The listing builds one solid part. Answer for the finished solid, in the listing's coordinates (mm). Face numbers are marked on the shaded views. A direction names the side the tool comes from. Coordinates: 2 decimals unless noted, no trailing zeros. Loops run counter-clockwise (first coordinate to the right, second up) from the corner with the lowest first, then second, coordinate; pieces in that order, holes last. Notation, with made-up numbers: (-17.75, -4.75) - (32.25, -4.75) arc R9 cw to (32.25, 8.25) - close; hole circle Ø4 at (6.5, 50.25). An arc over 180 degrees is marked (long way). Return JSON: item names as keys, results as strings. Group by question number.
1. Section C-C (y = -2.5) is taken. Write down the section's boundary in (x, z), and give its area (3 significant figures).
2. The mould has two halves that part along Z. Classify the marked faces 1, 2 and 3: pulls with the +Z half, pulls with the -Z half, needs draft (parallel to the pull), parting line crosses it, or undercut.
3. Section A-A (y = -27) is taken. Write down the section's boundary in (x, z), and give its area (3 significant figures).
4. Section D-D (y = 5.5) is taken. Write down the section's boundary in (x, z), and give its area (3 significant figures).
5. Find the intervals of material crossed by line 1 along Z through (x, y) = (0, -26.25); line 2 along X through (y, z) = (-17, 0); line 3 along Y through (x, z) = (0, -0.5), in increasing order.
6. Each of these flat-tipped pins is pushed along its axis until it touches: P1, Ø6, axis at x = 4.5, z = 7, coming from the +Y side; P2, Ø4, axis at x = -6.5, z = 8, coming from the +Y side; P3, Ø2, axis at x = -6.5, z = -5, coming from the +Y side. Where does it stop, or does it pass through?
7. Section B-B (x = 0) is taken. Write down the section's boundary in (y, z).
8. Which of the six approach directions +Z, -Z, +X, -X, +Y, -Y give full straight-line access (tool end or side, diameter ignored) to the marked faces 4, 5 and 6?
```python
from build123d import *

# Parameters (mm, degrees)
CROQUIS1_R              = 6.5
SALIENTE_EXTRUIR1_DEPTH = 12.5
CROQUIS3_W              = 19
CROQUIS3_H              = 25
CROQUIS3_R              = 6.5
SALIENTE_EXTRUIR2_DEPTH = 25
CROQUIS8_W              = 2
CROQUIS8_H              = 5


with BuildPart() as part:
    # Croquis1 → Saliente-Extruir1 (new body, symmetric)
    with BuildSketch(Plane.XY):
        with BuildLine():
            Line((-9.5, -10), (9.5, -10))
            Line((9.5, -10), (9.5, 0))
            ThreePointArc((9.5, 0), (0, 9.5), (-9.5, 0))
            Line((-9.5, 0), (-9.5, -10))
        make_face()
        Circle(CROQUIS1_R, mode=Mode.SUBTRACT)
    extrude(amount=SALIENTE_EXTRUIR1_DEPTH, both=True)

    # Croquis3 → Saliente-Extruir2 (add)
    with BuildSketch(Plane(origin=(0, -10, 0), x_dir=(-1, 0, 0), z_dir=(0, -1, 0))):
        Rectangle(CROQUIS3_W, CROQUIS3_H)
        Circle(CROQUIS3_R, mode=Mode.SUBTRACT)
    extrude(amount=SALIENTE_EXTRUIR2_DEPTH)

    # Croquis8 → Cortar-Revolución1 (revolve, cut)
    with BuildSketch(Plane.XY):
        Polygon((-11.434596491, -17.257283371), (-11.434596491, -12.257283371), (-9.5, -11.75), (-9.5, -16.75), align=None)
        with Locations((-10.5, -27.25)):
            Rectangle(CROQUIS8_W, CROQUIS8_H)
    revolve(axis=Axis((0, -6.5, 0), (0, -1, 0)), mode=Mode.SUBTRACT)


solid = part.part
```
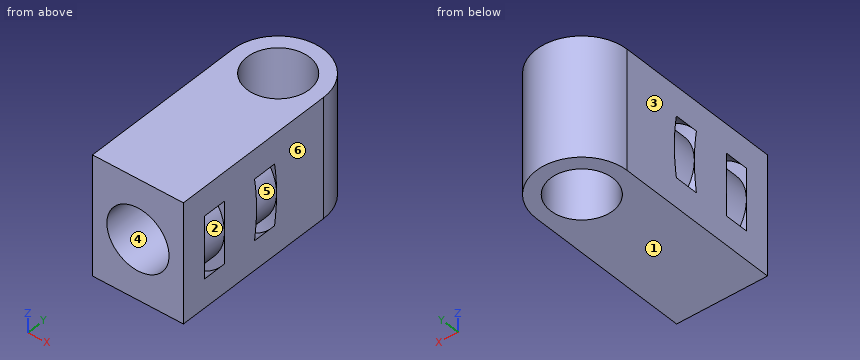
The answers:
{
 "1": {"outline": "(-9.5, -12.5) - (-6, -12.5) - (-6, 12.5) - (-9.5, 12.5) - close; (6, -12.5) - (9.5, -12.5) - (9.5, 12.5) - (6, 12.5) - close", "area": "175 mm2"},
 "2": {"face 1": "pulls with the -Z half", "face 2": "undercut", "face 3": "needs draft"},
 "3": {"outline": "(-9.5, -12.5) - (9.5, -12.5) - (9.5, -6.48) arc R11.5 cw to (-9.5, -6.48) - close; circle Ø19 at (0, 0); (-9.5, 6.48) arc R11.5 cw to (9.5, 6.48) - (9.5, 12.5) - (-9.5, 12.5) - close; hole circle Ø13 at (0, 0)", "area": "246 mm2"},
 "4": {"outline": "(-7.75, -12.5) - (-3.46, -12.5) - (-3.46, 12.5) - (-7.75, 12.5) - close; (3.46, -12.5) - (7.75, -12.5) - (7.75, 12.5) - (3.46, 12.5) - close", "area": "214 mm2"},
 "5": {"line 1": "z = -12.5 to -11.5, -9.5 to -6.5, 6.5 to 9.5, 11.5 to 12.5", "line 2": "x = -9.5 to -6.5, 6.5 to 9.5", "line 3": "y = -10 to -6.5, 6.5 to 9.5"},
 "6": {"P1": "stops at y = 9.38", "P2": "stops at y = 8.37", "P3": "stops at y = 7.75"},
 "7": {"outline": "(-35, -12.5) - (-6.5, -12.5) - (-6.5, 12.5) - (-35, 12.5) - (-35, 6.5) - (-10, 6.5) - (-10, -6.5) - (-35, -6.5) - close; (6.5, -12.5) - (9.5, -12.5) - (9.5, 12.5) - (6.5, 12.5) - close; hole (-29.75, -11.5) - (-24.75, -11.5) - (-24.75, -9.5) - (-29.75, -9.5) - close; hole (-29.75, 9.5) - (-24.75, 9.5) - (-24.75, 11.5) - (-29.75, 11.5) - close; hole (-17.26, -11.43) - (-12.26, -11.43) - (-11.75, -9.5) - (-16.75, -9.5) - close; hole (-17.26, 11.43) - (-16.75, 9.5) - (-11.75, 9.5) - (-12.26, 11.43) - close"},
 "8": {"face 4": "-Y", "face 5": "none", "face 6": "+Z, -Z, +X, +Y, -Y"}
}
